from build123d import *

# Parameters (mm, degrees)
SKETCH1_R           = 26.67
BOSS_EXTRUDE1_DEPTH = 3.175


with BuildPart() as part:
    # Sketch1 → Boss-Extrude1 (new body)
    with BuildSketch(Plane.XY):
        Circle(SKETCH1_R)
        with BuildLine():
            ThreePointArc((-2.175224917, 1.9685), (-2.9337, 0), (-2.175224917, -1.9685))
            Line((-2.175224917, -1.9685), (2.175224917, -1.9685))
            ThreePointArc((2.175224917, -1.9685), (2.9337, 0), (2.175224917, 1.9685))
            Line((2.175224917, 1.9685), (-2.175224917, 1.9685))
        make_face(mode=Mode.SUBTRACT)
    extrude(amount=BOSS_EXTRUDE1_DEPTH)


solid = part.part
The model under review builds one solid part; all positions refer to its coordinate system, in mm. A direction names the side the tool comes from. Round coordinates to 2 decimals unless told otherwise and drop trailing zeros. Order: outer loops, then holes, each group sorted by start corner. A loop starts at its lowest first (then second) coordinate and runs counter-clockwise, first axis right, second up. Notation, with made-up numbers: (68.25, 87.25) -> (77.25, 87.25) arc R17 ccw to (77.25, 117.25) -> close; hole circle Ø9 at (86.25, 57). An arc over 180 degrees is marked (long way). Return JSON: item names as keys, results as strings.
1. The part is to be moulded in two halves that separate along X. For faces 1 (the face through (0, -6, 0)), 2 (the face through (0, -1.968, 2)), 3 (the face through (-3.472, 26.443, 1.565)), say which applies: +X half, -X half, draft (parallel to the pull), parting line (faces both ways), or undercut.
Answer block:
{"face 1": "draft", "face 2": "undercut", "face 3": "parting line"}
2. Insertion check: P1, Ø1, axis at x = 14, z = 2.5, coming from the -Y side; P2, Ø1.6, axis at x = 0, z = 2, coming from the -Y side. Each pin has a flat end and moves straight along its axis. Give the tip position at first contact, or say it passes through.
Answer block:
{"P1": "stops at y = -23", "P2": "stops at y = -26.67"}
3. For L1, parallel to Y at x = -1.5, z = 0.5; L2, parallel to X at y = -11, z = 0.6; L3, parallel to X at y = 13, z = 1.65, list the stretches that pass through material, from the lowest coordinate up. Write a range as [from, to].
Answer block:
{"L1": "y = [-26.63, -1.97], [1.97, 26.63]", "L2": "x = [-24.3, 24.3]", "L3": "x = [-23.29, 23.29]"}
4. Take a section at A-A (x = 0). Write out the cut boundary in (y, z) (1 decimal).
Answer block:
{"outline": "(-26.7, 0) -> (-2, 0) -> (-2, 3.2) -> (-26.7, 3.2) -> close; (2, 0) -> (26.7, 0) -> (26.7, 3.2) -> (2, 3.2) -> close"}
5. Take a section at C-C (z = 1.25). Write out the cut boundary in (x, y).
Answer block:
{"outline": "circle Ø53.34 at (0, 0); hole (-2.18, -1.97) -> (2.18, -1.97) arc R2.93 ccw to (2.18, 1.97) -> (-2.18, 1.97) arc R2.93 ccw to start"}
6. Take a section at D-D (x = -20). Write out the cut boundary in (y, z) (3 decimals), then the cut area to 3 significant figures.
Answer block:
{"outline": "(-17.643, 0) -> (17.643, 0) -> (17.643, 3.175) -> (-17.643, 3.175) -> close", "area": "112 mm²"}
7. Take a section at B-B (y = 0). Write out the cut boundary in (x, z) (3 decimals).
Answer block:
{"outline": "(-26.67, 0) -> (-2.934, 0) -> (-2.934, 3.175) -> (-26.67, 3.175) -> close; (2.934, 0) -> (26.67, 0) -> (26.67, 3.175) -> (2.934, 3.175) -> close"}
8. For faces 4 (the face through (2.934, -0.03, 1.565)), 5 (the face through (0, -6, 3.175)), list the 3-axis set-ups (+Z, -Z, +X, -X, +Y, -Y) from which the entire face can be reached by the end or side of a thin tool; tool diameter is ignored.
Answer block:
{"face 4": "+Z, -Z", "face 5": "+Z, +X, -X, +Y, -Y"}
